Can you work these out from the model? Positions are in its coordinate system, mm. A direction names the side the tool comes from. Round coordinates to 2 decimals unless told otherwise and drop trailing zeros. Order: outer loops, then holes, each group sorted by start corner. A loop starts at its lowest first (then second) coordinate and runs counter-clockwise, first axis right, second up. Notation, with made-up numbers: (79, -10) - (133, -10) arc R13 cw to (133, 12) - close; hole circle Ø9 at (-0.5, 53). An arc over 180 degrees is marked (long way). Write item = value, one per line.
from build123d import *

# Parameters (mm, degrees)
BASE_W                                           = 342.9
BASE_H                                           = 508
BOSS_EXTRUDE1_DEPTH                              = 25.4
SKETCH2_W                                        = 406.4
SKETCH2_H                                        = 25.4
CUT_EXTRUDE1_DEPTH                               = 10.16
CBORE_FOR_3_8_SOCKET_HEAD_CAP_SCREW4_D           = 9.8044
CBORE_FOR_3_8_SOCKET_HEAD_CAP_SCREW4_DEPTH       = 15.24
CBORE_FOR_3_8_SOCKET_HEAD_CAP_SCREW4_CBORE_D     = 15.875
CBORE_FOR_3_8_SOCKET_HEAD_CAP_SCREW4_CBORE_DEPTH = 9.525
CBORE_FOR_3_8_SOCKET_HEAD_CAP_SCREW3_D           = 9.8044
CBORE_FOR_3_8_SOCKET_HEAD_CAP_SCREW3_DEPTH       = 25.4
CBORE_FOR_3_8_SOCKET_HEAD_CAP_SCREW3_CBORE_D     = 15.875
CBORE_FOR_3_8_SOCKET_HEAD_CAP_SCREW3_CBORE_DEPTH = 15.24
CBORE_FOR_1_4_SOCKET_HEAD_CAP_SCREW1_D           = 6.5278
CBORE_FOR_1_4_SOCKET_HEAD_CAP_SCREW1_DEPTH       = 25.4
CBORE_FOR_1_4_SOCKET_HEAD_CAP_SCREW1_CBORE_D     = 11.1125
CBORE_FOR_1_4_SOCKET_HEAD_CAP_SCREW1_CBORE_DEPTH = 6.35
CUT_EXTRUDE3_DEPTH                               = 12.7
SKETCH10_W                                       = 6.35
SKETCH10_H                                       = 457.2
SKETCH10_W_2                                     = 292.1
SKETCH10_H_2                                     = 6.35
CUT_EXTRUDE4_DEPTH                               = 6.35
F_3_8_16_TAPPED_HOLE2_D                          = 7.9375
F_3_8_16_TAPPED_HOLE2_DEPTH                      = 25.4
SKETCH19_R                                       = 9.525
CUT_EXTRUDE5_DEPTH                               = 1.27


with BuildPart() as part:
    # Base → Boss-Extrude1 (new body)
    with BuildSketch(Plane(origin=(0, 0, 0), x_dir=(1, 0, 0), z_dir=(0, 1, 0))):
        with Locations((-30.52641196, -120.249169435)):
            Rectangle(BASE_W, BASE_H)
    extrude(amount=BOSS_EXTRUDE1_DEPTH)

    # Sketch2 → Cut-Extrude1 (cut)
    with BuildSketch(Plane(origin=(0, 25.4, 0), x_dir=(1, 0, 0), z_dir=(0, 1, 0))):
        with Locations((-30.52641196, -44.049169435)):
            Rectangle(SKETCH2_W, SKETCH2_H)
    extrude(amount=-CUT_EXTRUDE1_DEPTH, mode=Mode.SUBTRACT)

    # CBORE for 3/8 Socket Head Cap Screw4
    with Locations(Plane(origin=(83.77358804, 0, 44.049169435), x_dir=(0, 0, -1), z_dir=(0, -1, 0))):
        with Locations((0, 0), (0, -114.3), (0, -228.6)):
            CounterBoreHole(CBORE_FOR_3_8_SOCKET_HEAD_CAP_SCREW4_D / 2, CBORE_FOR_3_8_SOCKET_HEAD_CAP_SCREW4_CBORE_D / 2, CBORE_FOR_3_8_SOCKET_HEAD_CAP_SCREW4_CBORE_DEPTH, depth=CBORE_FOR_3_8_SOCKET_HEAD_CAP_SCREW4_DEPTH)

    # CBORE for 3/8 Socket Head Cap Screw3
    with Locations(Plane(origin=(0, 0, 0), x_dir=(-1, 0, 0), z_dir=(0, -1, 0))):
        with Locations((-113.93608804, -71.989169435), (-113.93608804, -112.629169435), (174.98891196, -71.989169435), (174.98891196, -112.629169435)):
            CounterBoreHole(CBORE_FOR_3_8_SOCKET_HEAD_CAP_SCREW3_D / 2, CBORE_FOR_3_8_SOCKET_HEAD_CAP_SCREW3_CBORE_D / 2, CBORE_FOR_3_8_SOCKET_HEAD_CAP_SCREW3_CBORE_DEPTH, depth=CBORE_FOR_3_8_SOCKET_HEAD_CAP_SCREW3_DEPTH)

    # CBORE for 1/4 Socket Head Cap Screw1
    with Locations(Plane(origin=(128.22358804, 0, 361.549169435), x_dir=(0, 0, -1), z_dir=(0, -1, 0))):
        with Locations((0, 0), (0, -317.5), (482.6, -317.5), (482.6, 0)):
            CounterBoreHole(CBORE_FOR_1_4_SOCKET_HEAD_CAP_SCREW1_D / 2, CBORE_FOR_1_4_SOCKET_HEAD_CAP_SCREW1_CBORE_D / 2, CBORE_FOR_1_4_SOCKET_HEAD_CAP_SCREW1_CBORE_DEPTH, depth=CBORE_FOR_1_4_SOCKET_HEAD_CAP_SCREW1_DEPTH)

    # Sketch8 → Cut-Extrude3 (cut)
    with BuildSketch(Plane(origin=(0, 25.4, 0), x_dir=(1, 0, 0), z_dir=(0, 1, 0))):
        with BuildLine():
            Line((140.92358804, -374.249169435), (115.52358804, -374.249169435))
            Line((115.52358804, -374.249169435), (115.52358804, -356.469169435))
            add(Edge.make_bspline(
                [(115.52358804, -356.469169435), (115.52358804, -353.916782548), (115.309325815, -351.653056376), (114.148772711, -349.642919435)],
                knots=[0, 0, 0, 0, 1, 1, 1, 1], degree=3))
            ThreePointArc((114.148772711, -349.642919435), (114.401056025, -347.72663742), (116.31733804, -347.474354107))
            add(Edge.make_bspline(
                [(123.14358804, -348.849169435), (120.822481832, -348.849169435), (118.327474981, -348.634907211), (116.31733804, -347.474354107)],
                knots=[0, 0, 0, 0, 1, 1, 1, 1], degree=3))
            Line((123.14358804, -348.849169435), (140.92358804, -348.849169435))
            Line((140.92358804, -348.849169435), (140.92358804, -374.249169435))
        make_face()
        with BuildLine():
            Line((-201.97641196, -374.249169435), (-176.57641196, -374.249169435))
            Line((-176.57641196, -374.249169435), (-176.57641196, -356.469169435))
            add(Edge.make_bspline(
                [(-175.201596632, -349.642919435), (-176.794150567, -352.401303766), (-176.57641196, -354.968722974), (-176.57641196, -356.469169435)],
                knots=[0, 0, 0, 0, 1, 1, 1, 1], degree=3))
            ThreePointArc((-175.201596632, -349.642919435), (-175.453879945, -347.72663742), (-177.37016196, -347.474354107))
            add(Edge.make_bspline(
                [(-177.37016196, -347.474354107), (-180.128546291, -349.066908042), (-182.695965499, -348.849169435), (-184.19641196, -348.849169435)],
                knots=[0, 0, 0, 0, 1, 1, 1, 1], degree=3))
            Line((-184.19641196, -348.849169435), (-201.97641196, -348.849169435))
            Line((-201.97641196, -348.849169435), (-201.97641196, -374.249169435))
        make_face()
        with BuildLine():
            Line((-201.97641196, 133.750830565), (-176.57641196, 133.750830565))
            Line((-176.57641196, 133.750830565), (-176.57641196, 115.970830565))
            add(Edge.make_bspline(
                [(-176.57641196, 115.970830565), (-176.57641196, 113.418443678), (-176.362149736, 111.154717506), (-175.201596632, 109.144580565)],
                knots=[0, 0, 0, 0, 1, 1, 1, 1], degree=3))
            ThreePointArc((-175.201596632, 109.144580565), (-175.453879945, 107.22829855), (-177.37016196, 106.976015236))
            add(Edge.make_bspline(
                [(-177.37016196, 106.976015236), (-179.380298901, 108.13656834), (-181.875305752, 108.350830565), (-184.19641196, 108.350830565)],
                knots=[0, 0, 0, 0, 1, 1, 1, 1], degree=3))
            Line((-184.19641196, 108.350830565), (-201.97641196, 108.350830565))
            Line((-201.97641196, 108.350830565), (-201.97641196, 133.750830565))
        make_face()
        with BuildLine():
            Line((140.92358804, 133.750830565), (115.52358804, 133.750830565))
            Line((115.52358804, 133.750830565), (115.52358804, 115.970830565))
            add(Edge.make_bspline(
                [(114.148772711, 109.144580565), (115.309325815, 111.154717506), (115.52358804, 113.649724357), (115.52358804, 115.970830565)],
                knots=[0, 0, 0, 0, 1, 1, 1, 1], degree=3))
            ThreePointArc((114.148772711, 109.144580565), (114.401056025, 107.22829855), (116.31733804, 106.976015236))
            add(Edge.make_bspline(
                [(123.14358804, 108.350830565), (120.822481832, 108.350830565), (118.327474981, 108.13656834), (116.31733804, 106.976015236)],
                knots=[0, 0, 0, 0, 1, 1, 1, 1], degree=3))
            Line((123.14358804, 108.350830565), (140.92358804, 108.350830565))
            Line((140.92358804, 108.350830565), (140.92358804, 133.750830565))
        make_face()
    extrude(amount=-CUT_EXTRUDE3_DEPTH, mode=Mode.SUBTRACT)

    # Sketch10 → Cut-Extrude4 (cut)
    with BuildSketch(Plane(origin=(0, 25.4, 0), x_dir=(1, 0, 0), z_dir=(0, 1, 0))):
        with Locations((128.22358804, -120.249169435)):
            Rectangle(SKETCH10_W, SKETCH10_H)
        with Locations((-189.27641196, -120.249169435)):
            Rectangle(SKETCH10_W, SKETCH10_H)
        with Locations((-30.52641196, 121.050830565)):
            Rectangle(SKETCH10_W_2, SKETCH10_H_2)
        with Locations((-30.52641196, -361.549169435)):
            Rectangle(SKETCH10_W_2, SKETCH10_H_2)
    extrude(amount=-CUT_EXTRUDE4_DEPTH, mode=Mode.SUBTRACT)

    # 3/8-16 Tapped Hole2
    with Locations(Plane(origin=(0, 0, 0), x_dir=(-1, 0, 0), z_dir=(0, -1, 0))):
        with Locations((-107.90358804, -341.229169435), (168.95641196, -341.229169435), (168.95641196, 100.730830565), (-107.90358804, 100.730830565)):
            Hole(F_3_8_16_TAPPED_HOLE2_D / 2, depth=F_3_8_16_TAPPED_HOLE2_DEPTH)

    # Sketch19 → Cut-Extrude5 (cut)
    with BuildSketch(Plane.XZ):
        with Locations((-168.95641196, -100.730830565)):
            Circle(SKETCH19_R)
        with Locations((-168.95641196, 341.229169435)):
            Circle(SKETCH19_R)
        with Locations((107.90358804, 341.229169435)):
            Circle(SKETCH19_R)
        with Locations((108.217263786, -100.730830565)):
            Circle(SKETCH19_R)
    extrude(amount=-CUT_EXTRUDE5_DEPTH, mode=Mode.SUBTRACT)


solid = part.part
(1) On a 3-axis mill with a long thin cutter (end or side, diameter ignored), from which of +Z, -Z, +X, -X, +Y, -Y can I reach the whole of each face in a straight line? I mean faces 4 (the face through (-33, 20, 31.349)), 5 (the face through (88.634, 12.423, 43.411)), 6 (the face through (-176.576, 19, 365)), 7 (the face through (108, 1.27, -105)). Say none if no direction works.
Computed:
face_4 = +X, -X, +Y
face_5 = +Y, -Y
face_6 = +Z, -X, +Y
face_7 = -Y
(2) Will these pins go through, and if not, where does the flat tip stop? P1, Ø5, axis at x = -162.5, z = 63, coming from the -Y side; P2, Ø10, axis at x = 128.22, z = 361.55, coming from the -Y side; P3, Ø11.5, axis at x = 107.9, z = 341.23, coming from the -Y side; P4, Ø8, axis at x = 116.5, z = 111, coming from the -Y side.
Computed:
P1 = 0
P2 = 6.35
P3 = 1.27
P4 = 15.24
(3) Thinking about a two-plate mould opening in Z: for faces 1 (the face through (-197, 25.4, -39)), 2 (the face through (-193, 19, -108.351)), 3 (the face through (-192, 6.35, 359)), which applies, +Z half, -Z half, draft (parallel to the pull), parting line (faces both ways), or undercut?
Computed:
face_1 = draft
face_2 = -Z half
face_3 = undercut
(4) If I drill on line 1 (X direction, y = 21, z = 166.5); line 2 (Z direction, x = 23, y = 19.75); line 3 (X direction, y = 21.75, z = 111), over which ranges is the centre line in solid material (lowest first)? Write a range as from..to.
Computed:
line_1 = -201.98..-192.45, -186.1..125.05, 131.4..140.92
line_2 = -133.75..-124.23, -117.88..31.35, 56.75..358.37, 364.72..374.25
line_3 = -201.98..-192.45, -186.1..-179.61, -170.37..109.31, 118.56..125.05, 131.4..140.92
(5) If we section it at A-A (x = -71): Write out the boundary of the cut face in (y, z).
Computed:
outline = (0, -133.75) - (25.4, -133.75) - (25.4, -124.23) - (19.05, -124.23) - (19.05, -117.88) - (25.4, -117.88) - (25.4, 31.35) - (15.24, 31.35) - (15.24, 56.75) - (25.4, 56.75) - (25.4, 358.37) - (19.05, 358.37) - (19.05, 364.72) - (25.4, 364.72) - (25.4, 374.25) - (0, 374.25) - close
